Autodesk Inventor part; units mm, degrees
ref_plane "YZ Plane" through (0, 0, 0) normal (1, 0, 0) x (0, 1, 0)
ref_plane "XZ Plane" through (0, 0, 0) normal (0, 1, 0) x (-1, 0, 0)
ref_plane "XY Plane" through (0, 0, 0) normal (0, 0, 1) x (1, 0, 0)
sketch "Esboço1" plane through (0, 0, 0) normal (0, 1, 0) x (-1, 0, 0)
  line L0 (0.0003, 60.0007) -> (0.0003, 29.9998)
  line L1 (0.0003, 29.9998) -> (0.0003, 29.9999)
  line L2 (-0.9997, 29.9999) -> (-0.9997, 60.0007)
  line L3 (0.0003, 29.9999) -> (0.0003, 14.4635)
  line L4 (-0.9997, 14.4635) -> (-0.9997, 29.9999)
  line L5 (44.5003, 33.7635) -> (45.5003, 33.7635)
  line L6 (44.5003, 58.1254) -> (45.5003, 58.1254)
  line L7 (26.2003, 33.7635) -> (26.2003, 37.2635)
  line L8 (26.2003, 37.2635) -> (44.5003, 37.2635)
  line L9 (22.2003, 33.7635) -> (0.0003, 33.7635)
  line L10 (22.2003, 33.7635) -> (22.2003, 37.2635)
  line L11 (26.2003, 33.7635) -> (45.0003, 33.7635)
  line L12 (37.268, 41.2635) -> (44.5003, 41.2635)
  line L13 (22.2003, 37.2635) -> (26.2003, 41.2635)
  line L14 (37.268, 41.2635) -> (26.2003, 41.2635)
  line L15 (43.0622, 54.6254) -> (44.5003, 54.6254)
  line L16 (43.0622, 54.6254) -> (26.2003, 54.6254)
  line L17 (26.2003, 54.6254) -> (26.2003, 58.1254)
  line L18 (22.2003, 54.6254) -> (22.2503, 58.1254)
  line L19 (26.2003, 50.6254) -> (22.2003, 54.6254)
  line L20 (26.2003, 50.6254) -> (44.5003, 50.6254)
  line L21 (0.0003, 58.1254) -> (22.2503, 58.1254)
  line L22 (26.2003, 58.1254) -> (44.5003, 58.1254)
  line L23 (44.5003, 54.6254) -> (44.5003, 58.1254)
  line L24 (44.5003, 48.0257) -> (44.5003, 50.6254)
  line L25 (44.5003, 33.7635) -> (44.5003, 37.2635)
  line L26 (44.5003, 41.2635) -> (44.5003, 45.0257)
  line L27 (44.5003, 37.2635) -> (44.5003, 41.2635)
  line L28 (44.5003, 45.0257) -> (44.5003, 48.0257)
  line L29 (44.5003, 50.6254) -> (44.5003, 54.6254)
  line L30 (44.5003, 33.968) -> (44.5003, 11.768)
  line L31 (44.5003, 11.768) -> (0.0003, 11.768)
  line L32 (0.0003, 11.768) -> (0.0003, 14.4635)
  line L33 (45.5003, 33.7635) -> (45.5003, 11.768)
  line L34 (44.5003, 58.1254) -> (44.5003, 77.4254)
  line L35 (44.5003, 77.4254) -> (0.0003, 77.4254)
  line L36 (0.0003, 60.0007) -> (0.0003, 77.4254)
  line L37 (45.5003, 58.1254) -> (45.5003, 77.4254)
  line L38 (45.5003, 77.4254) -> (44.5003, 78.4254)
  line L39 (0.0003, 78.4254) -> (-0.9997, 77.4254)
  line L40 (0.0003, 78.4254) -> (44.5003, 78.4254)
  line L41 (-0.9997, 60.0007) -> (-0.9997, 77.4254)
  line L42 (0.0003, 10.768) -> (-0.9997, 11.768)
  line L43 (45.5003, 11.768) -> (44.5003, 10.768)
  line L44 (-0.9997, 11.768) -> (-0.9997, 14.4635)
  line L45 (0.0003, 10.768) -> (44.5003, 10.768)
  line L46 (4.3192, 41.5257) -> (5.3003, 41.5257)
  line L47 (4.8098, 51.5257) -> (5.3003, 51.5257)
  line L48 (5.3003, 41.5257) -> (5.3003, 51.5257)
  line L49 (4.3192, 41.5257) -> (0.0003, 41.5257)
  line L50 (4.8098, 51.5257) -> (0.0003, 51.5257)
  point P0 (0, 0)
  dimension "d40" = 1
  dimension "d86" = 44.5
  dimension "d90" = 1
  dimension "d91" = 1
  dimension "d94" = 4
  dimension "d116" = 22.2
  dimension "d118" = 19.3
extrude "Extrusão30" add sketch "Esboço1" along normal blind 6 contours L36 L35 L34 L22 L17 L16 L15 L29 L20 L19 L18 L21 L0 | L50 L47 L48 L46 L49 L0 | L9 L10 L13 L14 L12 L27 L8 L7 L11 L30 L31 L32 L3 L0
extrude "Extrusão32" add sketch "Esboço1" along normal blind 18 contours L21 L18 L19 L20 L24 L28 L26 L12 L14 L13 L10 L9 L0 L49 L46 L48 L47 L50 | L23 L15 L16 L17 L22 | L11 L7 L8 L25
extrude "Extrusão33" add sketch "Esboço1" along normal blind 7 contours L0 L3 L32 L31 L30 L5 L33 L43 L45 L42 L44 L4 L2 L41 L39 L40 L38 L37 L6 L34 L35 L36
sketch "Esboço4" plane through (0, 0, 0) normal (0, -1, 0) x (1, 0, 0)
  line L0 (-44.5003, 11.768) -> (-0.0003, 11.768)
  line L1 (-0.0003, 77.4254) -> (-44.5003, 77.4254)
  line L2 (-44.5003, 33.7635) -> (-44.5003, 58.1254)
  line L3 (-0.0003, 41.5257) -> (-0.0003, 51.5257)
  circle A0 centre (-22.2503, 44.5969) radius 3.75
  line L4 (-26.2003, 58.1254) -> (-26.2003, 54.6254)
  line L5 (-22.2503, 58.1254) -> (-0.0003, 58.1254)
  arc A1 (-20.3067, 58.1254) -> (-24.2503, 58.5969) centre (-22.2503, 58.5969) ccw
  arc A2 (-24.2003, 30.597) -> (-20.2003, 30.597) centre (-22.2003, 30.597) ccw
  line L6 (-22.2003, 33.7635) -> (-0.0003, 33.7635)
  line L7 (-24.2003, 30.597) -> (-24.6441, 41.7103)
  line L8 (-20.2003, 30.597) -> (-19.853, 41.7132)
  line L9 (-24.2503, 58.5969) -> (-24.6458, 47.4821)
  line L10 (-20.2503, 58.5969) -> (-19.8549, 47.4821)
  point P0 (0, 0)
  point P1 (-20.2336, 58.1254)
  dimension "d141" = 7.5
  dimension "d155" = 4
  dimension "d156" = 4
extrude "Extrusão35" cut sketch "Esboço4" against normal blind 3 contours A0 | A0 L9 A1 L5 L10 | L8 A2 L7 A0
properties part number "Suporte"
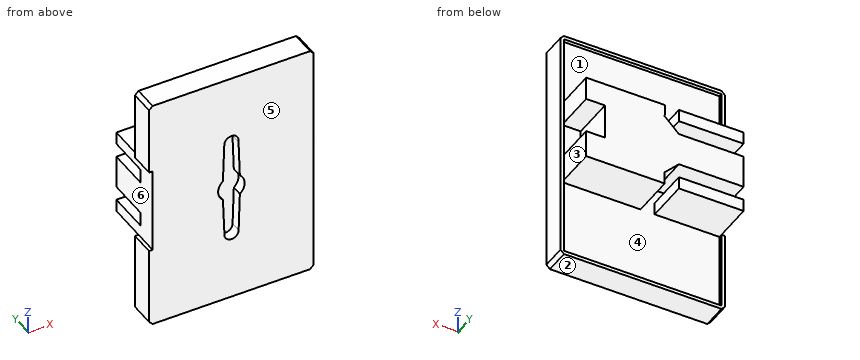
Input: part model. Units: mm. Frame: model coordinates. Face numbers are marked on the shaded views. A direction names the side the tool comes from. Coordinates: 2 decimals unless noted, no trailing zeros. Loops run counter-clockwise (first coordinate to the right, second up) from the corner with the lowest first, then second, coordinate; pieces in that order, holes last. Notation, with made-up numbers: M 76.5,47 L 107.5,47 A16 cw 107.5,64 Z; hole C 75.5,-20 d1. An arc over 180 degrees is marked long. Use a Markdown table: item, result. Add a question column.
1) Line query: L1, parallel to Z at x = -33, y = 8; L2, parallel to X at y = 4, z = 48; L3, parallel to X at y = 1, z = 59. Output: solid intervals per line, ascending. Write a range as from..to.
2) Draft query along X for the marked faces 1, 2, 3 and 4. Return one class per face: +X half, -X half, draft (parallel to the pull), parting line (faces both ways), or undercut.
3) Set-up query: the marked faces 5 and 6. Return all of +Z, -Z, +X, -X, +Y, -Y with unobstructed straight access to the full face (end or side cutting, diameter ignored); none if empty.
4) Section C-C, the plane z = 24. Return the cut outline in (x, y), plus the area to 3 significant figures.
5) Section A-A, the plane y = 11.25. Return the cut outline in (x, z), plus the area to 3 significant figures.
6) Section B-B, the plane x = -8. Return the cut outline in (y, z), plus the area to 3 significant figures.
7) Section D-D, the plane x = -2.5. Return the cut outline in (y, z), plus the area to 3 significant figures.
8) Pin query (flat end, axial travel): P1, Ø0.8, axis at x = -45, y = 3.5, coming from the -Z side; P2, Ø1.8, axis at y = 14.5, z = 56.5, coming from the +X side; P3, Ø1.6, axis at x = -1.5, y = 12.5, coming from the -Z side. Return the tip coordinate at first contact, or that it passes through.
Answer below:
| question | item | result |
|---|---|---|
| 1 | L1 | 33.76..37.26, 41.26..50.63, 54.63..58.13 |
| 1 | L2 | -44.5..1 |
| 1 | L3 | -45.5..-24.21, -20.29..1 |
| 2 | face 1 | undercut |
| 2 | face 2 | draft |
| 2 | face 3 | +X half |
| 2 | face 4 | undercut |
| 3 | face 5 | +Z, -Z, +X, -X, -Y |
| 3 | face 6 | -X, +Y, -Y |
| 4 | outline | M -45.5,0 L 1,0 L 1,7 L 0,7 L 0,6 L -44.5,6 L -44.5,7 L -45.5,7 Z |
| 4 | area | 281 mm2 |
| 5 | outline | M -44.5,33.76 L -26.2,33.76 L -26.2,37.26 L -44.5,37.26 Z; M -44.5,41.26 L -26.2,41.26 L -22.2,37.26 L -22.2,33.76 L 0,33.76 L 0,41.53 L -5.3,41.53 L -5.3,51.53 L 0,51.53 L 0,58.13 L -22.25,58.13 L -22.2,54.63 L -26.2,50.63 L -44.5,50.63 Z; M -44.5,54.63 L -26.2,54.63 L -26.2,58.13 L -44.5,58.13 Z |
| 5 | area | 841 mm2 |
| 6 | outline | M 0,10.77 L 7,10.77 L 7,11.77 L 6,11.77 L 6,33.76 L 18,33.76 L 18,58.13 L 6,58.13 L 6,77.43 L 7,77.43 L 7,78.43 L 0,78.43 Z |
| 6 | area | 700 mm2 |
| 7 | outline | M 0,10.77 L 7,10.77 L 7,11.77 L 6,11.77 L 6,33.76 L 18,33.76 L 18,41.53 L 6,41.53 L 6,51.53 L 18,51.53 L 18,58.13 L 6,58.13 L 6,77.43 L 7,77.43 L 7,78.43 L 0,78.43 Z |
| 7 | area | 580 mm2 |
| 8 | P1 | z = 10.87 |
| 8 | P2 | x = 0 |
| 8 | P3 | z = 33.76 |
